CAD build for the part. Positions are in the model's coordinates, mm. Coordinates: 2 decimals unless noted, no trailing zeros. Loops run counter-clockwise (first coordinate to the right, second up) from the corner with the lowest first, then second, coordinate; pieces in that order, holes last. Notation, with made-up numbers: (2.25, 35.5) -> (22.25, 35.5) arc R15 cw to (22.25, 45.5) -> close; hole circle Ø7 at (-2.5, 60.5). An arc over 180 degrees is marked (long way). Return JSON: item names as keys, results as strings. Group by question number.
(1) Saw through at B-B on y = 1.05. Give the number of separate pieces and of enclosed holes in the cut face, then the cut area to 3 significant figures.
(2) Saw through at C-C on z = -15.5. Write the cut outline in (x, y).
(3) Mould opens along Z. For faces 1 (the face through (-1, 0, -1)), 2 (the face through (-70.14, 1.48, -15.98)) say: pulls with the +Z half, pulls with the -Z half, needs draft (parallel to the pull), parting line crosses it, or undercut.
(4) Flat gauge pins, fed straight in: pin 1 Ø0.9 at (y, z) = (2, 25.5) entering from +X; pin 2 Ø0.6 at (y, z) = (1, 21.5) entering from -X. Where does each tip first touch, or does it go through?
(5) Saw through at A-A on z = 42.5. Write the cut outline in (x, y).
(6) Probe L1, parallel to X at y = 1.95, z = -22 (3 decimals); L2, parallel to X at y = 1.05, z = -64; L3, parallel to Z at x = 10.5, y = 1.5. List the from-to ranges inside material, lowest first.
```python
from build123d import *

# Parameters (mm, degrees)
SKETCH1_W           = 120
SKETCH1_H           = 140
BOSS_EXTRUDE1_DEPTH = 3
SKETCH2_R           = 1.5
CUT_EXTRUDE1_DEPTH  = 107.343782141
SKETCH3_2_R         = 1.5
CUT_EXTRUDE3_DEPTH  = 107.343782141
SKETCH3_R           = 1.5
CUT_EXTRUDE2_DEPTH  = 107.343782141
SKETCH4_R           = 1.5
CUT_EXTRUDE4_DEPTH  = 107.343782141
SKETCH5_R           = 1.5
CUT_EXTRUDE5_DEPTH  = 3
SKETCH6_R           = 1.525
SKETCH6_W           = 10
SKETCH6_H           = 2.05
SKETCH6_W_2         = 20
CUT_EXTRUDE7_DEPTH  = 107.343782141
SKETCH9_R           = 1.525
CUT_EXTRUDE8_DEPTH  = 3
SKETCH10_W          = 44
SKETCH10_H          = 12
CUT_EXTRUDE9_DEPTH  = 5
SKETCH11_R          = 1.5
CUT_EXTRUDE10_DEPTH = 5


with BuildPart() as part:
    # Sketch1 → Boss-Extrude1 (new body)
    with BuildSketch(Plane(origin=(0, 0, 0), x_dir=(1, 0, 0), z_dir=(0, 1, 0))):
        Rectangle(SKETCH1_W, SKETCH1_H)
        Polygon((-80, 21.791828604), (-60, 10), (-60, 70), (-80, 70), align=None)
        Polygon((80, 70), (60, 70), (60, 10), (80, 21.791828604), align=None)
    extrude(amount=BOSS_EXTRUDE1_DEPTH)

    # Sketch2 → Cut-Extrude1 (cut, through all)
    with BuildSketch(Plane(origin=(0, 3, 0), x_dir=(1, 0, 0), z_dir=(0, 1, 0))):
        with Locations(Location((-38, -60, 0), (0, 0, 270))):
            Circle(SKETCH2_R)
        with Locations(Location((-25, -27, 0), (0, 0, 270))):
            Circle(SKETCH2_R)
        with Locations(Location((5, -27, 0), (0, 0, 270))):
            Circle(SKETCH2_R)
        with Locations(Location((-8, -60, 0), (0, 0, 270))):
            Circle(SKETCH2_R)
        with Locations(Location((35, -27, 0), (0, 0, 270))):
            Circle(SKETCH2_R)
        with Locations(Location((22, -60, 0), (0, 0, 270))):
            Circle(SKETCH2_R)
    extrude(amount=-CUT_EXTRUDE1_DEPTH, mode=Mode.SUBTRACT)

    # Sketch3<2> → Cut-Extrude3 (cut, through all)
    with BuildSketch(Plane(origin=(0, 3, 0), x_dir=(1, 0, 0), z_dir=(0, 1, 0))):
        with Locations(Location((-27.529579069, 60.385555627, 0), (0, 0, 270))):
            Circle(SKETCH3_2_R)
        with Locations(Location((-27.529579069, 7.385555627, 0), (0, 0, 90))):
            Circle(SKETCH3_2_R)
        with Locations(Location((27.470420931, 7.385555627, 0), (0, 0, 270))):
            Circle(SKETCH3_2_R)
        with Locations(Location((27.470420931, 60.385555627, 0), (0, 0, 90))):
            Circle(SKETCH3_2_R)
    extrude(amount=-CUT_EXTRUDE3_DEPTH, mode=Mode.SUBTRACT)

    # Sketch3 → Cut-Extrude2 (cut, through all)
    with BuildSketch(Plane(origin=(0, 3, 0), x_dir=(1, 0, 0), z_dir=(0, 1, 0))):
        with Locations(Location((-27.529579069, 60.385555627, 0), (0, 0, 270))):
            Circle(SKETCH3_R)
        with Locations(Location((-27.529579069, 7.385555627, 0), (0, 0, 90))):
            Circle(SKETCH3_R)
        with Locations(Location((27.470420931, 7.385555627, 0), (0, 0, 270))):
            Circle(SKETCH3_R)
        with Locations(Location((27.470420931, 60.385555627, 0), (0, 0, 90))):
            Circle(SKETCH3_R)
    extrude(amount=-CUT_EXTRUDE2_DEPTH, mode=Mode.SUBTRACT)

    # Sketch4 → Cut-Extrude4 (cut, through all)
    with BuildSketch(Plane(origin=(0, 3, 0), x_dir=(1, 0, 0), z_dir=(0, 1, 0))):
        with Locations(Location((-75, 34.863883517, 0), (0, 0, 270))):
            Circle(SKETCH4_R)
        with Locations(Location((-75, 58.863883517, 0), (0, 0, 270))):
            Circle(SKETCH4_R)
        with Locations(Location((-46, 34.863883517, 0), (0, 0, 90))):
            Circle(SKETCH4_R)
        with Locations(Location((-46, 58.863883517, 0), (0, 0, 90))):
            Circle(SKETCH4_R)
        with Locations(Location((46, 58.863883517, 0), (0, 0, 270))):
            Circle(SKETCH4_R)
        with Locations(Location((46, 34.863883517, 0), (0, 0, 270))):
            Circle(SKETCH4_R)
        with Locations(Location((75, 34.863883517, 0), (0, 0, 90))):
            Circle(SKETCH4_R)
        with Locations(Location((75, 58.863883517, 0), (0, 0, 90))):
            Circle(SKETCH4_R)
    extrude(amount=-CUT_EXTRUDE4_DEPTH, mode=Mode.SUBTRACT)

    # Sketch5 → Cut-Extrude5 (cut)
    with BuildSketch(Plane(origin=(0, 3, 0), x_dir=(1, 0, 0), z_dir=(0, 1, 0))):
        with Locations(Location((-68, 30, 0), (0, 0, 270))):
            Circle(SKETCH5_R)
        with Locations(Location((-53, 30, 0), (0, 0, 270))):
            Circle(SKETCH5_R)
    extrude(amount=-CUT_EXTRUDE5_DEPTH, mode=Mode.SUBTRACT)

    # Sketch6 → Cut-Extrude7 (cut, through all)
    with BuildSketch(Plane(origin=(0, 3, 0), x_dir=(1, 0, 0), z_dir=(0, 1, 0))):
        with Locations(Location((-53, -64.8, 0), (0, 0, 270))):
            Circle(SKETCH6_R)
        with Locations(Location((53, -64.8, 0), (0, 0, 90))):
            Circle(SKETCH6_R)
        with Locations((-40, -53.975)):
            Rectangle(SKETCH6_W, SKETCH6_H)
        with Locations((40, -53.975)):
            Rectangle(SKETCH6_W, SKETCH6_H)
        with Locations((30, -21.725)):
            Rectangle(SKETCH6_W_2, SKETCH6_H)
        with Locations((-30, -21.725)):
            Rectangle(SKETCH6_W_2, SKETCH6_H)
        with Locations((35, 23.325)):
            Rectangle(SKETCH6_W, SKETCH6_H)
        with Locations((-35, 23.325)):
            Rectangle(SKETCH6_W, SKETCH6_H)
    extrude(amount=-CUT_EXTRUDE7_DEPTH, mode=Mode.SUBTRACT)

    # Sketch9 → Cut-Extrude8 (cut)
    with BuildSketch(Plane(origin=(0, 3, 0), x_dir=(1, 0, 0), z_dir=(0, 1, 0))):
        with Locations(Location((-54, 22, 0), (0, 0, 270))):
            Circle(SKETCH9_R)
        with Locations(Location((54, 22, 0), (0, 0, 90))):
            Circle(SKETCH9_R)
    extrude(amount=-CUT_EXTRUDE8_DEPTH, mode=Mode.SUBTRACT)

    # Sketch10 → Cut-Extrude9 (cut)
    with BuildSketch(Plane(origin=(0, 3, 0), x_dir=(1, 0, 0), z_dir=(0, 1, 0))):
        with Locations((0.046472237, -6.975074484)):
            Rectangle(SKETCH10_W, SKETCH10_H)
    extrude(amount=-CUT_EXTRUDE9_DEPTH, mode=Mode.SUBTRACT)

    # Sketch11 → Cut-Extrude10 (cut)
    with BuildSketch(Plane(origin=(0, 3, 0), x_dir=(1, 0, 0), z_dir=(0, 1, 0))):
        with Locations(Location((-53, 64, 0), (0, 0, 270))):
            Circle(SKETCH11_R)
        with Locations(Location((53, 64, 0), (0, 0, 270))):
            Circle(SKETCH11_R)
    extrude(amount=-CUT_EXTRUDE10_DEPTH, mode=Mode.SUBTRACT)


solid = part.part
```
Geometry results:
{
 "1": {"separate pieces": "1", "enclosed holes": "33", "area": "18,100 mm²"},
 "2": {"outline": "(-69.33, 0) -> (69.33, 0) -> (69.33, 3) -> (-69.33, 3) -> close"},
 "3": {"face 1": "needs draft", "face 2": "pulls with the +Z half"},
 "4": {"pin 1": "x = 60", "pin 2": "x = -60"},
 "5": {"outline": "(-60, 0) -> (60, 0) -> (60, 3) -> (-60, 3) -> close"},
 "6": {"L1": "-80 to -55.525, -52.475 to 52.475, 55.525 to 80", "L2": "-80 to -54.5, -51.5 to 51.5, 54.5 to 80", "L3": "-70 to 0.98, 12.98 to 70"}
}
